Design review of the part built by this model. Coordinates are the model's own, in mm. Face numbers are marked on the shaded views. Coordinates: 2 decimals unless noted, no trailing zeros. Write each loop counter-clockwise with the first axis right and the second up, starting at its lowest first coordinate (ties: lowest second). Pieces come first, ordered by that corner, then holes. Notation, with made-up numbers: (1, -34.5) - (54, -34.5) arc R8 cw to (54, -26.5) - close; hole circle Ø6 at (68, -18.75). An arc over 180 degrees is marked (long way). Answer as CSV lines item,"result". Start each with the question number.
Q1. Clearance check with flat-ended pins moving along their axes: pin 1 (20.5 mm diameter, centred on x = -7.5, z = -14, fed in from -Y); pin 2 (24 mm diameter, centred on x = 4.5, y = -58.5, fed in from +Z); pin 3 (3 mm diameter, centred on y = -132.5, z = -34, fed in from -X). State where each tip first meets the part, or that it passes through.
Q2. We need section A-A (z = 0). Write out the cut boundary in (x, y).
Q3. We need section C-C (x = 0). Write out the cut boundary in (y, z), plus the area to 3 significant figures.
Q4. For line 1 along Z through (x, y) = (10.5, -167.5); line 2 along X through (y, z) = (-124, -37); line 3 along Y through (x, z) = (18, -11), list the stretches that pass through material, from the lowest coordinate up. Write a range as [from, to].
Q5. We need section B-B (y = -170). Write out the cut boundary in (x, z), plus the area to 3 significant figures.
Q6. We need section D-D (z = -25.5). Write out the cut boundary in (x, y).
Q7. Mouldability with a two-part tool opening along X and no side actions: class the marked faces 1 and 2 as pulls with the +X half, pulls with the -X half, needs draft (parallel to the pull), parting line crosses it, or undercut.
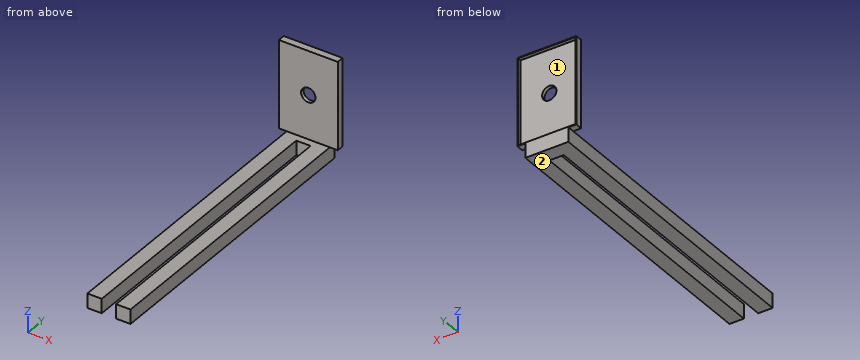
from build123d import *

# Parameters (mm, degrees)
SKETCH1_W           = 40
SKETCH1_H           = 60
SKETCH1_R           = 5
BOSS_EXTRUDE1_DEPTH = 2.5
SKETCH2_W           = 41
SKETCH2_H           = 61
SKETCH2_W_2         = 40
SKETCH2_H_2         = 60
BOSS_EXTRUDE2_DEPTH = 5
SKETCH3_W           = 30
SKETCH3_H           = 10
BOSS_EXTRUDE3_DEPTH = 10
SKETCH4_W           = 10
SKETCH4_H           = 10
BOSS_EXTRUDE4_DEPTH = 200


with BuildPart() as part:
    # Sketch1 → Boss-Extrude1 (new body)
    with BuildSketch(Plane(origin=(0, 0, 0), x_dir=(1, 0, 0), z_dir=(0, 1, 0))):
        Rectangle(SKETCH1_W, SKETCH1_H)
        with Locations(Location((0, 0, 0), (0, 0, 270))):
            Circle(SKETCH1_R, mode=Mode.SUBTRACT)
    extrude(amount=BOSS_EXTRUDE1_DEPTH)

    # Sketch2 → Boss-Extrude2 (add)
    with BuildSketch(Plane.XZ):
        Rectangle(SKETCH2_W, SKETCH2_H)
        Rectangle(SKETCH2_W_2, SKETCH2_H_2, mode=Mode.SUBTRACT)
    extrude(amount=-BOSS_EXTRUDE2_DEPTH)

    # Sketch3 → Boss-Extrude3 (add)
    with BuildSketch(Plane(origin=(0, 0, -30.5), x_dir=(-1, 0, 0), z_dir=(0, 0, -1))):
        Rectangle(SKETCH3_W, SKETCH3_H)
    extrude(amount=BOSS_EXTRUDE3_DEPTH)

    # Sketch4 → Boss-Extrude4 (add)
    with BuildSketch(Plane.XZ.offset(5)):
        with Locations((-10, -35.5)):
            Rectangle(SKETCH4_W, SKETCH4_H)
        with Locations((10, -35.5)):
            Rectangle(SKETCH4_W, SKETCH4_H)
    extrude(amount=BOSS_EXTRUDE4_DEPTH)


solid = part.part
Results list:
1,pin 1,"stops at y = 0"
1,pin 2,"stops at z = -30.5"
1,pin 3,"stops at x = -15"
2,outline,"(-20.5, 0) - (-5, 0) - (-5, 2.5) - (-20, 2.5) - (-20, 5) - (-20.5, 5) - close; (5, 0) - (20.5, 0) - (20.5, 5) - (20, 5) - (20, 2.5) - (5, 2.5) - close"
3,outline,"(-5, -40.5) - (5, -40.5) - (5, -30) - (2.5, -30) - (2.5, -5) - (0, -5) - (0, -30.5) - (-5, -30.5) - close; (0, 5) - (2.5, 5) - (2.5, 30) - (5, 30) - (5, 30.5) - (0, 30.5) - close"
3,area,"230 mm2"
4,line 1,"z = [-40.5, -30.5]"
4,line 2,"x = [-15, -5], [5, 15]"
4,line 3,"y = [0, 2.5]"
5,outline,"(-15, -40.5) - (-5, -40.5) - (-5, -30.5) - (-15, -30.5) - close; (5, -40.5) - (15, -40.5) - (15, -30.5) - (5, -30.5) - close"
5,area,"200 mm2"
6,outline,"(-20.5, 0) - (20.5, 0) - (20.5, 5) - (20, 5) - (20, 2.5) - (-20, 2.5) - (-20, 5) - (-20.5, 5) - close"
7,face 1,"undercut"
7,face 2,"needs draft"
